```python
from build123d import *

# Parameters (mm, degrees)
BOSS_EXTRUDE2_DEPTH = 74.676
SHELL1_T            = -3.175
BOSS_EXTRUDE3_REACH = 101.695
SKETCH7_W           = 19.05
SKETCH7_H           = 41.37312771
SKETCH7_R           = 3.175
SKETCH7_H_2         = 29.549685012
BOSS_EXTRUDE4_DEPTH = 3.175


with BuildPart() as part:
    # Sketch4 → Boss-Extrude2 (new body)
    with BuildSketch(Plane(origin=(0, 0, 0), x_dir=(0, 0, -1), z_dir=(1, 0, 0))):
        Polygon((-44.915630504, 37.043578511), (78.274369496, 37.043578511), (57.954369496, -18.785162652), (57.954369496, -69.585162652), (-24.595630504, -69.585162652), (-24.595630504, -18.785162652), align=None)
    extrude(amount=BOSS_EXTRUDE2_DEPTH)

    # Shell1
    shell1_openings = [part.faces().sort_by_distance(p)[0] for p in [
        (37.338, 37.043578511, -16.679369496),
        (37.338, -69.585162652, -16.679369496),
    ]]
    offset(amount=SHELL1_T, openings=shell1_openings, kind=Kind.INTERSECTION)

    # Sketch6 → Boss-Extrude3 (add, up to next)
    with BuildSketch(Plane(origin=(0, 0, 21.420630504), x_dir=(-1, 0, 0), z_dir=(0, 0, -1)), mode=Mode.PRIVATE) as boss_extrude3_sk1:
        Polygon((-4.030024393, -18.785162652), (-25.4, -69.585162652), (-22.225, -69.585162652), (0, -18.785162652), align=None)
    boss_extrude3_tool1 = extrude(boss_extrude3_sk1.sketch, amount=BOSS_EXTRUDE3_REACH, mode=Mode.PRIVATE) - part.part
    add(boss_extrude3_tool1.solids().sort_by_distance((12.482636, -43.180418, 21.420631))[0])

    # Sketch7 → Boss-Extrude4 (add)
    with BuildSketch(Plane(origin=(0, 0, -57.954369496), x_dir=(-1, 0, 0), z_dir=(0, 0, -1))):
        with Locations((-65.151, -74.298598797)):
            Rectangle(SKETCH7_W, SKETCH7_H)
        with Locations((-65.151, -88.635162652)):
            Circle(SKETCH7_R, mode=Mode.SUBTRACT)
        with Locations((-9.525, -68.867228229)):
            Rectangle(SKETCH7_W, SKETCH7_H_2)
        with Locations((-9.525, -77.292070735)):
            Circle(SKETCH7_R, mode=Mode.SUBTRACT)
    boss_extrude4 = extrude(amount=BOSS_EXTRUDE4_DEPTH)

    # Mirror1: Boss-Extrude4 across plane
    add(boss_extrude4.mirror(Plane(origin=(0, 0, -16.679369496), x_dir=(1, 0, 0), z_dir=(0, 0, -1))))


solid = part.part
```
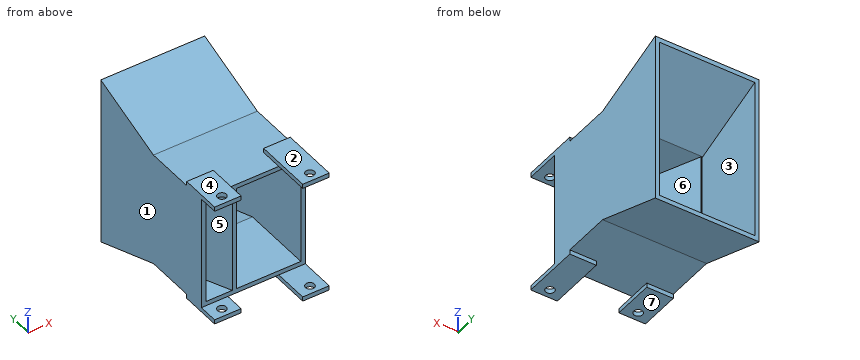
Can you work these out from the model? Positions are in its coordinate system, mm. Face numbers are marked on the shaded views. A direction names the side the tool comes from. Round coordinates to 2 decimals unless told otherwise and drop trailing zeros. Loops run counter-clockwise (first coordinate to the right, second up) from the corner with the lowest first, then second, coordinate; pieces in that order, holes last. Notation, with made-up numbers: (85, -24.5) -> (143, -24.5) arc R14 cw to (143, -9.5) -> close; hole circle Ø6 at (-16, 41). An arc over 180 degrees is marked (long way). Answer in a Markdown table with one row per item.
Item 1: Suppose I cut it at C-C, the plane y = 25. List the corners of the cut face in (x, z) for me (3 decimals).
Answer block:
| item | result |
|---|---|
| outline | (0, -73.891) -> (74.676, -73.891) -> (74.676, 40.532) -> (0, 40.532) -> close; hole (3.175, -70.512) -> (71.501, -70.512) -> (71.501, 37.153) -> (3.175, 37.153) -> close |
Item 2: On a 3-axis mill with a long thin cutter (end or side, diameter ignored), from which of +Z, -Z, +X, -X, +Y, -Y can I reach the whole of each face in a straight line? I mean the marked faces 4, 5, 6 and 7. Say none if no direction works.
Answer block:
| item | result |
|---|---|
| face 4 | +Z, +X, -X, -Y |
| face 5 | -Y |
| face 6 | +Y |
| face 7 | -Z, +X, -X, -Y |
Item 3: If I drill on probe 1 along X at (y, z) = (21, -49) (3 decimals); probe 2 along Z at (x, y) = (12.5, -23); probe 3 along X at (y, z) = (-26.5, -27.5) (3 decimals), over which ranges is the centre line in solid material (lowest first)?
Answer block:
| item | result |
|---|---|
| probe 1 | 0 to 3.175, 71.501 to 74.676 |
| probe 2 | -57.95 to -54.78, 21.42 to 24.6 |
| probe 3 | 0 to 3.175, 3.375 to 7.275, 71.501 to 74.676 |
Item 4: Suppose I cut it at A-A, the plane z = -0.5. List the corners of the cut face in (x, y) for me (3 decimals).
Answer block:
| item | result |
|---|---|
| outline | (0, -69.585) -> (3.175, -69.585) -> (3.175, -26.042) -> (22.225, -69.585) -> (25.4, -69.585) -> (4.03, -18.785) -> (3.175, -18.785) -> (3.175, 37.044) -> (0, 37.044) -> close; (71.501, -69.585) -> (74.676, -69.585) -> (74.676, 37.044) -> (71.501, 37.044) -> close |
Item 5: We'd pull the mould along X, two halves only. Please class the marked faces 1, 2 and 3: released by +X, released by -X, zero draft, split by the parting line, or undercut.
Answer block:
| item | result |
|---|---|
| face 1 | released by -X |
| face 2 | zero draft |
| face 3 | undercut |
Item 6: Suppose I cut it at D-D, the plane x = 59.5. List the corners of the cut face in (y, z) for me, plus the area to 3 significant figures.
Answer block:
| item | result |
|---|---|
| outline | (-94.99, -61.13) -> (-53.61, -61.13) -> (-53.61, -57.95) -> (-18.79, -57.95) -> (37.04, -78.27) -> (37.04, -74.9) -> (-18.23, -54.78) -> (-69.59, -54.78) -> (-69.59, -57.95) -> (-94.99, -57.95) -> close; (-94.99, 24.6) -> (-69.59, 24.6) -> (-69.59, 21.42) -> (-18.23, 21.42) -> (37.04, 41.54) -> (37.04, 44.92) -> (-18.79, 24.6) -> (-53.61, 24.6) -> (-53.61, 27.77) -> (-94.99, 27.77) -> close |
| area | 962 mm² |
Item 7: Suppose I cut it at B-B, the plane x = 48.5. List the corners of the cut face in (y, z) for me.
Answer block:
| item | result |
|---|---|
| outline | (-69.59, -57.95) -> (-18.79, -57.95) -> (37.04, -78.27) -> (37.04, -74.9) -> (-18.23, -54.78) -> (-69.59, -54.78) -> close; (-69.59, 21.42) -> (-18.23, 21.42) -> (37.04, 41.54) -> (37.04, 44.92) -> (-18.79, 24.6) -> (-69.59, 24.6) -> close |
Item 8: Will these pins go through, and if not, where does the flat tip stop? P1, Ø9.5, axis at x = 12, y = -72, coming from the -Z side; P2, Ø15, axis at x = 17, y = -49.5, coming from the +Z side; P3, Ø3, axis at x = 44.5, y = -11, coming from the -Z side.
Answer block:
| item | result |
|---|---|
| P1 | z = -61.13 |
| P2 | z = 27.77 |
| P3 | z = -61.33 |
